```python
from build123d import *

# Parameters (mm, degrees)
EXTRUDE_1_DEPTH = 17
EXTRUDE_2_DEPTH = 12
SKETCH_3_W      = 6
SKETCH_3_H      = 7
EXTRUDE_3_DEPTH = 12
SKETCH_4_W      = 10
SKETCH_4_H      = 33
EXTRUDE_4_DEPTH = 40
SKETCH_10_W     = 10
SKETCH_10_H     = 33
EXTRUDE_5_DEPTH = 10


with BuildPart() as part:
    # Sketch 2 → Extrude 1 (new body)
    with BuildSketch(Plane.XY):
        Polygon((-19.204371621, 15.843606587), (-19.204371621, -17.156393413), (20.795628379, -17.156393413), (-12.204371621, 15.843606587), align=None)
    extrude(amount=EXTRUDE_1_DEPTH)

    # Sketch 2_3 → Extrude 2 (add)
    with BuildSketch(Plane.XY):
        Polygon((0.911243772, 15.844973174), (-12.204371621, 15.843606587), (20.795628379, -17.156393413), (20.795628379, -6.156393413), (10.795628379, -6.156393413), (10.853436076, 1.344289881), (10.911243772, 8.844973174), (0.911243772, 8.844973174), align=None)
    extrude(amount=EXTRUDE_2_DEPTH)

    # Sketch 3 → Extrude 3 (add)
    with BuildSketch(Plane(origin=(20.795628379, 0, 0), x_dir=(0, 0, -1), z_dir=(1, 0, 0))):
        with Locations((-3, -2.656393413)):
            Rectangle(SKETCH_3_W, SKETCH_3_H)
    extrude(amount=-EXTRUDE_3_DEPTH)



with BuildPart() as body_2:
    # Sketch 4 → Extrude 4 (new body)
    with BuildSketch(Plane(origin=(20.795628379, 0, 0), x_dir=(0, 0, -1), z_dir=(1, 0, 0))):
        with Locations((5, -0.656393413)):
            Rectangle(SKETCH_4_W, SKETCH_4_H)
    extrude(amount=-EXTRUDE_4_DEPTH)


with BuildPart() as part_1:
    add(part.part)

    add(body_2.part)  # Extrude 5 merges body 2
    # Sketch 10 → Extrude 5 (add)
    with BuildSketch(Plane(origin=(20.795628379, 0, 0), x_dir=(0, 0, -1), z_dir=(1, 0, 0))):
        with Locations((5, -0.656393413)):
            Rectangle(SKETCH_10_W, SKETCH_10_H)
    extrude(amount=EXTRUDE_5_DEPTH)


solid = part_1.part
```
Can you work these out from the model? Positions are in its coordinate system, mm. A direction names the side the tool comes from. Give positions to 0.01 mm unless a question says otherwise; leave off trailing zeros. Loops run counter-clockwise (first coordinate to the right, second up) from the corner with the lowest first, then second, coordinate; pieces in that order, holes last. Notation, with made-up numbers: M -40,-14.75 L 11,-14.75 A19 ccw 11,-10.75 Z; hole C 6.5,81 d9. An arc over 180 degrees is marked long. Use one line per item in the form item = value. Start each with the question number.
(1) I want a section at B-B, the plane x = 12. Write out the boundary of the cut face in (y, z).
(2) I want a section at C-C, the plane y = -10.5. Write out the boundary of the cut face in (x, z), and give its area (3 significant figures).
(3) I want a section at A-A, the plane z = 11.25. Write out the boundary of the cut face in (x, y), and give its area (3 significant figures).
(4) On a 3-axis mill with a long thin cutter (end or side, diameter ignored), from which of +Z, -Z, +X, -X, +Y, -Y can I reach the whole of each face in a straight line? I mean faces 1 (the flat face through (20.796, -10, 5)), 2 (the flat face through (30.796, 0, -5)), 3 (the flat face through (6, 8.845, 6)). Say none if no direction works.
(5) I want a section at D-D, the plane z = 14.75. Write out the boundary of the cut face in (x, y).
(6) Please list where these lines run through material, in increasing order: line 1 (Y direction, x = 12, z = -2.5); line 2 (X direction, y = 13.5, z = 7); line 3 (Y direction, x = 11.5, z = 3.25).
(7) I'm going to push flat-ended pins straight in: P1, Ø2, axis at x = 15, y = -1.5, coming from the +Z side; P2, Ø1, axis at y = 0.5, z = 1.5, coming from the +X side; P3, Ø5, axis at x = 14.5, z = 3.5, coming from the +Y side. Where does each tip first touch, or does it pass through?
Worked out:
q1.outline = M -17.16,-10 L 15.84,-10 L 15.84,0 L 0.84,0 L 0.84,6 L -6.16,6 L -6.16,12 L -8.36,12 L -8.36,17 L -17.16,17 Z
q2.outline = M -19.2,-10 L 30.8,-10 L 30.8,0 L 20.8,0 L 20.8,12 L 14.14,12 L 14.14,17 L -19.2,17 Z
q2.area = 1,150 mm²
q3.outline = M -19.2,-17.16 L 20.8,-17.16 L 20.8,-6.16 L 10.8,-6.16 L 10.91,8.84 L 0.91,8.84 L 0.91,15.84 L -12.2,15.84 L -19.2,15.84 Z
q3.area = 1,030 mm²
q4.face_1 = +Z, +X, +Y, -Y
q4.face_2 = +Z, -Z, +X, +Y, -Y
q4.face_3 = +Z, +X, +Y
q5.outline = M -19.2,-17.16 L 20.8,-17.16 L -12.2,15.84 L -19.2,15.84 Z
q6.line_1 = -17.16 to 15.84
q6.line_2 = -19.2 to 0.91
q6.line_3 = -17.16 to 0.84
q7.P1 = 6
q7.P2 = 20.8
q7.P3 = 0.84
